from build123d import *

# Parameters (mm, degrees)
CONG_1_R = 10
CONG_2_R = 1


with BuildPart() as part:
    # Esquisse1 → Révolution2 (revolve)
    with BuildSketch(Plane.XY):
        with BuildLine():
            Line((-12.5, 28.2), (-12.5, 31.5))
            Line((-12.5, 31.5), (-9.5, 31.5))
            Line((-9.5, 31.5), (-9.5, 34.5))
            Line((-9.5, 34.5), (-12.5, 34.5))
            Line((-12.5, 34.5), (-12.5, 37.8))
            Line((-12.5, 37.8), (0, 37.8))
            Line((0, 37.8), (0, 95.8))
            ThreePointArc((0, 95.8), (-6.891439137, 91.863012013), (-7, 83.927016654))
            Line((-7, 83.927016654), (-15.5, 41.8))
            Line((-15.5, 41.8), (-15.5, 25.2))
            Line((-15.5, 25.2), (-12.5, 25.2))
            Line((-12.5, 25.2), (-9.5, 25.2))
            Line((-9.5, 25.2), (-9.5, 28.2))
            Line((-9.5, 28.2), (-12.5, 28.2))
        make_face()
    revolve(axis=Axis((0, 95.8, 0), (0, -1, 0)))

    # Congé1
    cong_1_edges = [part.edges().sort_by_distance(p)[0] for p in [
        (15.5, 41.8, 0),
        (7, 83.927016654, 0),
    ]]
    fillet(cong_1_edges, radius=CONG_1_R)

    # Congé2
    cong_2_edges = [part.edges().sort_by_distance(p)[0] for p in [
        (15.5, 25.2, 0),
    ]]
    fillet(cong_2_edges, radius=CONG_2_R)


solid = part.part
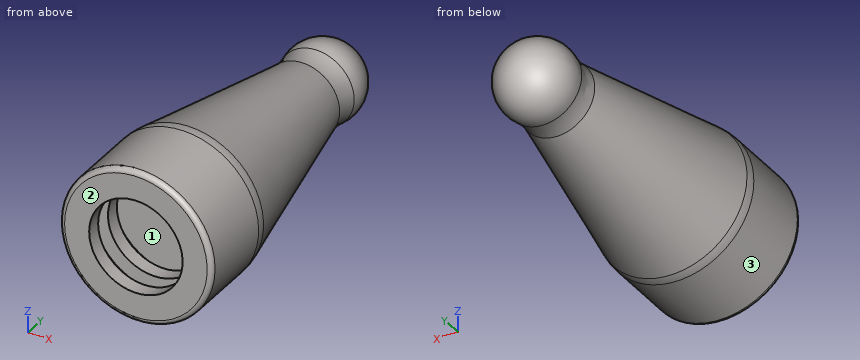
Design review of the part built by this model. Coordinates are the model's own, in mm. Face numbers are marked on the shaded views. Coordinates: 2 decimals unless noted, no trailing zeros. Write each loop counter-clockwise with the first axis right and the second up, starting at its lowest first coordinate (ties: lowest second). Pieces come first, ordered by that corner, then holes. Notation, with made-up numbers: (50, 1.25) - (100, 1.25) arc R25 cw to (100, 36.25) - close; hole circle Ø3 at (70.25, 36.5). An arc over 180 degrees is marked (long way). One line per item, written item: value.
1) Insertion check: pin 1 (8 mm diameter, centred on y = 40, z = -9, fed in from +X); pin 2 (7.5 mm diameter, centred on x = 4, z = 1.5, fed in from -Y); pin 3 (1 mm diameter, centred on y = 75.5, z = -5, fed in from +X). Each pin has a flat end and moves straight along its axis. Give the tip position at first contact, or say it passes through.
Answer sheet:
pin 1: stops at x = 14.67
pin 2: stops at y = 37.8
pin 3: stops at x = 7.47
2) Mouldability with a two-part tool opening along X and no side actions: class the marked faces 1, 2 and 3 as +X half, -X half, draft (parallel to the pull), parting line (faces both ways), or undercut.
Answer sheet:
face 1: undercut
face 2: draft
face 3: parting line
3) Add section A-A (y = 35.5). State the section outline as (x, z) points.
Answer sheet:
outline: circle Ø31 at (0, 0); hole circle Ø25 at (0, 0)
4) Add section B-B (y = 71.5). State the section outline as (x, z) points, plus the area to 3 significant figures.
Answer sheet:
outline: circle Ø19.01 at (0, 0)
area: 284 mm2
5) Add section C-C (y = 52). State the section outline as (x, z) points.
Answer sheet:
outline: circle Ø26.88 at (0, 0)
6) To check wall thickness, follow probe 1 along Z at (x, y) = (0, 30.2); probe 2 along X at (y, z) = (26.1, 0); probe 3 along Z at (x, y) = (0, 32.2). State the ranges of each line that lie inside material, in increasing order.
Answer sheet:
probe 1: z = -15.5 to -12.5, 12.5 to 15.5
probe 2: x = -15.49 to -9.5, 9.5 to 15.49
probe 3: z = -15.5 to -9.5, 9.5 to 15.5
